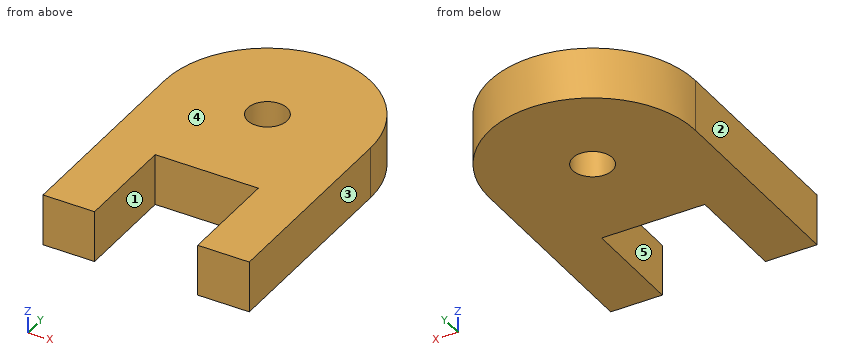
from build123d import *

# Parameters (mm, degrees)
SKETCH1_R           = 0.6096
BOSS_EXTRUDE1_DEPTH = 1.5875
SKETCH2_W           = 3.175
SKETCH2_H           = 3.175
CUT_EXTRUDE1_DEPTH  = 8.274838916


with BuildPart() as part:
    # Sketch1 → Boss-Extrude1 (new body)
    with BuildSketch(Plane.XY):
        with BuildLine():
            Line((-3.175, 0), (-3.175, -6.35))
            Line((-3.175, -6.35), (3.175, -6.35))
            Line((3.175, -6.35), (3.175, 0))
            ThreePointArc((3.175, 0), (0, 3.175), (-3.175, 0))
        make_face()
        Circle(SKETCH1_R, mode=Mode.SUBTRACT)
    extrude(amount=BOSS_EXTRUDE1_DEPTH)

    # Sketch2 → Cut-Extrude1 (cut, through all)
    with BuildSketch(Plane(origin=(0, 0, 0), x_dir=(-1, 0, 0), z_dir=(0, 0, -1))):
        with Locations((0, -4.7625)):
            Rectangle(SKETCH2_W, SKETCH2_H)
    extrude(amount=-CUT_EXTRUDE1_DEPTH, mode=Mode.SUBTRACT)


solid = part.part
Work out the finished part from the listing and answer in its coordinate system (mm). Face numbers are marked on the shaded views. A direction names the side the tool comes from. Give positions to 0.01 mm unless a question says otherwise; leave off trailing zeros. Order: outer loops, then holes, each group sorted by start corner. A loop starts at its lowest first (then second) coordinate and runs counter-clockwise, first axis right, second up. Notation, with made-up numbers: (-35.75, 6) -> (-26.75, 6) arc R28 cw to (-26.75, 27) -> close; hole circle Ø6 at (16, 40.5). An arc over 180 degrees is marked (long way). Answer as a JSON object with one key per item and string values. Group by question number.
1. Section D-D on y = 2.75 is taken. Determine the outline of the cut face in (x, z).
2. Section A-A on x = 0 is taken. Determine the outline of the cut face in (y, z) (1 decimal), plus the area to 3 significant figures.
3. A flat-ended cylindrical pin translates along its axis: pin 1 Ø0.5 at (x, z) = (-0.5, 0.5) entering from -Y (3 decimals). Find the tip coordinate at first contact, or state that the pin passes through.
4. Section C-C on x = 2.5 is taken. Determine the outline of the cut face in (y, z).
5. Consider line 1 along Y through (x, z) = (0, 0.9) (3 decimals); line 2 along X through (y, z) = (-5, 0.1) (1 decimal); line 3 along X through (y, z) = (-0.5, 0.7) (3 decimals). Determine where each line is inside the solid, lowest interval first. Write a range as [from, to].
6. A tool of negligible diameter and unlimited length cuts with its end or side. For the marked faces 1 and 2, from which of +Z, -Z, +X, -X, +Y, -Y can it reach the whole face along a straight path? Write none if from no direction.
7. The mould has two halves that part along X. Classify the marked faces 3, 4 and 5: released by +X, released by -X, zero draft, split by the parting line, or undercut.
Result sheet:
{
 "1": {"outline": "(-1.59, 0) -> (1.59, 0) -> (1.59, 1.59) -> (-1.59, 1.59) -> close"},
 "2": {"outline": "(-3.2, 0) -> (-0.6, 0) -> (-0.6, 1.6) -> (-3.2, 1.6) -> close; (0.6, 0) -> (3.2, 0) -> (3.2, 1.6) -> (0.6, 1.6) -> close", "area": "8.15 mm^2"},
 "3": {"pin 1": "stops at y = -3.175"},
 "4": {"outline": "(-6.35, 0) -> (1.96, 0) -> (1.96, 1.59) -> (-6.35, 1.59) -> close"},
 "5": {"line 1": "y = [-3.175, -0.61], [0.61, 3.175]", "line 2": "x = [-3.2, -1.6], [1.6, 3.2]", "line 3": "x = [-3.175, -0.349], [0.349, 3.175]"},
 "6": {"face 1": "+Z, -Z, -Y", "face 2": "+Z, -Z, -X, +Y, -Y"},
 "7": {"face 3": "released by +X", "face 4": "zero draft", "face 5": "undercut"}
}
